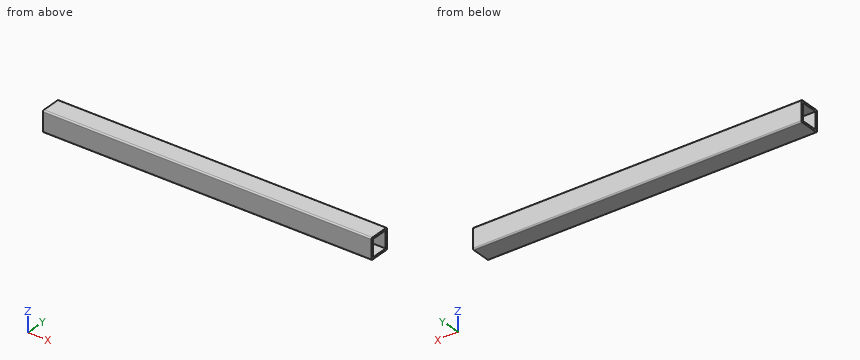
from build123d import *

# Parameters (mm, degrees)
F0_W     = 41.275
F0_H     = 41.275
F1_DEPTH = 400.05


with BuildPart() as f1:
    # F0 (on Right) → F1 (new body, symmetric)
    with BuildSketch(Plane.YZ):
        with BuildLine():
            ThreePointArc((25.4, 22.225), (24.470064, 24.470064), (22.225, 25.4))
            Line((22.225, 25.4), (-22.225, 25.4))
            ThreePointArc((-22.225, 25.4), (-24.470064, 24.470064), (-25.4, 22.225))
            Line((-25.4, 22.225), (-25.4, -22.225))
            ThreePointArc((-25.4, -22.225), (-24.470064, -24.470064), (-22.225, -25.4))
            Line((-22.225, -25.4), (22.225, -25.4))
            ThreePointArc((22.225, -25.4), (24.470064, -24.470064), (25.4, -22.225))
            Line((25.4, -22.225), (25.4, 22.225))
        make_face()
        Rectangle(F0_W, F0_H, mode=Mode.SUBTRACT)
    extrude(amount=F1_DEPTH, both=True)


solid = f1.part
Read the model definition and answer for the solid it produces. Units are mm, in the model's axes. Give positions to 0.01 mm unless a question says otherwise; leave off trailing zeros. Loops run counter-clockwise (first coordinate to the right, second up) from the corner with the lowest first, then second, coordinate; pieces in that order, holes last. Notation, with made-up numbers: (-15, 89) - (39, 89) arc R30 cw to (39, 123) - close; hole circle Ø8 at (52, 35.5). An arc over 180 degrees is marked (long way). Answer as CSV lines item,"result". Start each with the question number.
1) Straight lines are drawn through the part: L1, parallel to Z at x = 332, y = -5; L2, parallel to Z at x = -340, y = 23. For each, find the intervals that lie inside material, in ascending order. Write a range as from..to.
2) Find section A-A (y = -9). Write down the section's boundary in (x, z), then the cut area to 3 significant figures.
Findings below:
1,L1,"-25.4..-20.64, 20.64..25.4"
1,L2,"-25.3..25.3"
2,outline,"(-400.05, -25.4) - (400.05, -25.4) - (400.05, -20.64) - (-400.05, -20.64) - close; (-400.05, 20.64) - (400.05, 20.64) - (400.05, 25.4) - (-400.05, 25.4) - close"
2,area,"7,620 mm^2"
